```python
from build123d import *

# Parameters (mm, degrees)
SKETCH1_W                      = 19.05
SKETCH1_H                      = 25.4
BOSS_EXTRUDE1_DEPTH            = 38.1
TAP_DRILL_FOR_10_24_TAP1_D     = 3.7973
TAP_DRILL_FOR_10_24_TAP1_DEPTH = 19.05
TAP_DRILL_FOR_10_24_TAP1_TIP   = 1.140824014
SKETCH7_R                      = 9.525
CUT_EXTRUDE1_DEPTH             = 5.08


with BuildPart() as part:
    # Sketch1 → Boss-Extrude1 (new body)
    with BuildSketch(Plane.XY):
        with Locations((-9.525, 12.7)):
            Rectangle(SKETCH1_W, SKETCH1_H)
    extrude(amount=BOSS_EXTRUDE1_DEPTH)

    # Tap Drill for #10-24 Tap1
    with Locations(Plane.XY.offset(38.1)):
        with Locations((-10.583333333, 16.933333333), (-10.583333333, 8.466666667)):
            Hole(TAP_DRILL_FOR_10_24_TAP1_D / 2, depth=TAP_DRILL_FOR_10_24_TAP1_DEPTH)
            with Locations((0, 0, -(TAP_DRILL_FOR_10_24_TAP1_DEPTH + TAP_DRILL_FOR_10_24_TAP1_TIP / 2))):  # 118° drill point
                Cone(0, TAP_DRILL_FOR_10_24_TAP1_D / 2, TAP_DRILL_FOR_10_24_TAP1_TIP, mode=Mode.SUBTRACT)

    # Sketch7 → Cut-Extrude1 (cut)
    with BuildSketch(Plane(origin=(0, 0, 0), x_dir=(0, 0, -1), z_dir=(1, 0, 0))):
        with Locations(Location((-12.7, 12.7, 0), (0, 0, 90))):
            Circle(SKETCH7_R)
    extrude(amount=-CUT_EXTRUDE1_DEPTH, mode=Mode.SUBTRACT)


solid = part.part
```
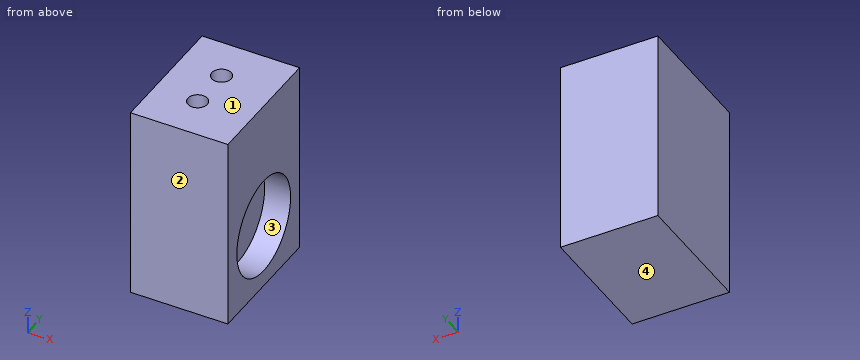
The listing builds one solid part. Answer for the finished solid, in the listing's coordinates (mm). Face numbers are marked on the shaded views. Give positions to 0.01 mm unless a question says otherwise; leave off trailing zeros. Order: outer loops, then holes, each group sorted by start corner. A loop starts at its lowest first (then second) coordinate and runs counter-clockwise, first axis right, second up.
Item 1: Given pin 1 Ø6 at (x, z) = (-4.5, 25) entering from -Y; pin 2 Ø5.5 at (y, z) = (9, 16.5) entering from +X, each flat-ended and moving along its own axis, determine where each tip first touches the part or whether it passes through.
From the geometry:
pin 1: stops at y = 0
pin 2: stops at x = -5.08
Item 2: Find the intervals of material crossed by probe 1 along X at (y, z) = (10.75, 21); probe 2 along Z at (x, y) = (-11.5, 7.25); probe 3 along X at (y, z) = (16, 34.5), in increasing order.
From the geometry:
probe 1: x = -19.05 to -5.08
probe 2: z = 0 to 18.82
probe 3: x = -19.05 to -12.24, -8.93 to 0
Item 3: The part is cut by section B-B, the plane z = 12.7. Give the vertices of the cut face in (x, y) (3 decimals), and give its area (3 significant figures).
From the geometry:
outline: (-19.05, 0) - (0, 0) - (0, 3.175) - (-5.08, 3.175) - (-5.08, 22.225) - (0, 22.225) - (0, 25.4) - (-19.05, 25.4) - close
area: 387 mm2
Item 4: The part is cut by section A-A, the plane y = 12.7. Give the vertices of the cut face in (x, z) (3 decimals).
From the geometry:
outline: (-19.05, 0) - (0, 0) - (0, 3.175) - (-5.08, 3.175) - (-5.08, 22.225) - (0, 22.225) - (0, 38.1) - (-19.05, 38.1) - close
Item 5: The part is cut by section C-C, the plane z = 34. Give the vertices of the cut face in (x, y), and give its area (3 significant figures).
From the geometry:
outline: (-19.05, 0) - (0, 0) - (0, 25.4) - (-19.05, 25.4) - close; hole circle Ø3.8 at (-10.58, 8.47); hole circle Ø3.8 at (-10.58, 16.93)
area: 461 mm2
Item 6: For a pull along Z with two mould halves and no side action, classify the marked faces 1, 2, 3 and 4 as pulls with the +Z half, pulls with the -Z half, needs draft (parallel to the pull), parting line crosses it, or undercut.
From the geometry:
face 1: pulls with the +Z half
face 2: needs draft
face 3: undercut
face 4: pulls with the -Z half
